Check sheet for the modelled part. Datum: model origin and axes. Units: mm. A direction names the side the tool comes from. Round coordinates to 2 decimals unless told otherwise and drop trailing zeros. Loops run counter-clockwise (first coordinate to the right, second up) from the corner with the lowest first, then second, coordinate; pieces in that order, holes last. Notation, with made-up numbers: M 46,19 L 50,19 A19 cw 50,48 Z; hole C 73,69 d9. An arc over 180 degrees is marked long. Write item = value, one per line. Start each with the question number.
(1) Set-up check for faces 1 (the face through (-19, 2, 0)), 2 (the face through (-18, 3, 13.61)): record each of +Z, -Z, +X, -X, +Y, -Y from which the full face is reachable in a straight line by a thin tool's end or side.
(2) Cross-section at D-D on z = 28. Record the boundary of the cut face in (x, y).
(3) Cross-section at A-A on x = -34. Record the boundary of the cut face in (y, z).
(4) Mould release check, pull along Z, two halves, no side actions. Record for faces 3 (the face through (-19, 2, 49.22)), 4 (the face through (-19, 0, 13)), 5 (the face through (-4.423, 2.535, 47.124)): pulls with the +Z half, pulls with the -Z half, needs draft (parallel to the pull), parting line crosses it, or undercut.
(5) Scan lines: L1, parallel to X at y = 2.8, z = 45.22; L2, parallel to Z at x = -14, y = 3.9; L3, parallel to Z at x = -34, y = 2.7. Record each from-to range of solid material in increasing order. Write a range as from..to.
(6) Cross-section at C-C on x = -21.5. Record the boundary of the cut face in (y, z), plus the area to 3 significant figures.
(7) Go/stop test with flat-tipped pins: P1, Ø2, axis at y = 1, z = 35.5, coming from the +X side; P2, Ø3, axis at x = -14, z = 45.22, coming from the -Y side. Record where each tip stops, or that it passes through.
(8) Cross-section at B-B on z = 45.22. Record the boundary of the cut face in (x, y).
from build123d import *

# Parameters (mm, degrees)
BOSS_EXTRUDE1_DEPTH = 5
SKETCH2_R           = 1.95
SKETCH2_W           = 22
SKETCH2_H           = 22
CUT_EXTRUDE1_DEPTH  = 6


with BuildPart() as part:
    # Sketch1 → Boss-Extrude1 (new body)
    with BuildSketch(Plane(origin=(0, 0, 0), x_dir=(1, 0, 0), z_dir=(0, 1, 0))):
        with BuildLine():
            Line((-36, 0), (-2, 0))
            ThreePointArc((-2, 0), (-0.585786438, -0.585786438), (0, -2))
            Line((0, -2), (0, -47.22))
            ThreePointArc((0, -47.22), (-0.585786438, -48.634213562), (-2, -49.22))
            Line((-2, -49.22), (-36, -49.22))
            ThreePointArc((-36, -49.22), (-37.414213562, -48.634213562), (-38, -47.22))
            Line((-38, -47.22), (-38, -2))
            ThreePointArc((-38, -2), (-37.414213562, -0.585786438), (-36, 0))
        make_face()
    extrude(amount=BOSS_EXTRUDE1_DEPTH)

    # Sketch2 → Cut-Extrude1 (cut, through all)
    with BuildSketch(Plane(origin=(0, 5, 0), x_dir=(1, 0, 0), z_dir=(0, 1, 0))):
        with Locations((-4, -4)):
            Circle(SKETCH2_R)
        with Locations((-14, -4)):
            Circle(SKETCH2_R)
        with Locations((-24, -4)):
            Circle(SKETCH2_R)
        with Locations((-54, -4)):
            Circle(SKETCH2_R)
        with Locations((-34, -4)):
            Circle(SKETCH2_R)
        with Locations((-44, -4)):
            Circle(SKETCH2_R)
        with Locations((-44, -45.22)):
            Circle(SKETCH2_R)
        with Locations((-34, -45.22)):
            Circle(SKETCH2_R)
        with Locations((-54, -45.22)):
            Circle(SKETCH2_R)
        with Locations((-24, -45.22)):
            Circle(SKETCH2_R)
        with Locations((-14, -45.22)):
            Circle(SKETCH2_R)
        with Locations((-4, -45.22)):
            Circle(SKETCH2_R)
        with Locations((-17.5, -24.61)):
            Rectangle(SKETCH2_W, SKETCH2_H)
    extrude(amount=-CUT_EXTRUDE1_DEPTH, mode=Mode.SUBTRACT)


solid = part.part
Result:
q1.face_1 = -Z, +X, -X, +Y, -Y
q1.face_2 = +Y, -Y
q2.outline = M -38,0 L -28.5,0 L -28.5,5 L -38,5 Z; M -6.5,0 L 0,0 L 0,5 L -6.5,5 Z
q3.outline = M 0,0 L 5,0 L 5,2.05 L 0,2.05 Z; M 0,5.95 L 5,5.95 L 5,43.27 L 0,43.27 Z; M 0,47.17 L 5,47.17 L 5,49.22 L 0,49.22 Z
q4.face_3 = pulls with the +Z half
q4.face_4 = needs draft
q4.face_5 = undercut
q5.L1 = -38..-35.95, -32.05..-25.95, -22.05..-15.95, -12.05..-5.95, -2.05..0
q5.L2 = 0..2.05, 5.95..13.61, 35.61..43.27, 47.17..49.22
q5.L3 = 0..2.05, 5.95..43.27, 47.17..49.22
q6.outline = M 0,0 L 5,0 L 5,13.61 L 0,13.61 Z; M 0,35.61 L 5,35.61 L 5,49.22 L 0,49.22 Z
q6.area = 136 mm^2
q7.P1 = 0
q7.P2 = through
q8.outline = M -38,0 L -35.95,0 L -35.95,5 L -38,5 Z; M -32.05,0 L -25.95,0 L -25.95,5 L -32.05,5 Z; M -22.05,0 L -15.95,0 L -15.95,5 L -22.05,5 Z; M -12.05,0 L -5.95,0 L -5.95,5 L -12.05,5 Z; M -2.05,0 L 0,0 L 0,5 L -2.05,5 Z
